```python
from build123d import *

# Parameters (mm, degrees)
F0_W         = 100
F0_H         = 100
F1_DEPTH     = 20
F2_T         = -1.6
F3_R         = 5
F4_T1_DEPTH  = 13.4
F4_S5_W      = 5
F4_S5_H      = 5
F4_T6_DEPTH  = 5
F4_S11_W     = 5
F4_S11_H     = 5
F4_T12_DEPTH = 5
F4_S17_W     = 5
F4_S17_H     = 5
F4_T18_DEPTH = 5
F4_S23_W     = 5
F4_S23_H     = 5
F4_T24_DEPTH = 5
F5_R         = 5
F6_R         = 5


# Not quite as in the source:
# - a fillet or chamfer that OpenCascade refuses, or shapes differently, is made with other operations: its cross-section is extruded or revolved along the edge and cut away or added


with BuildPart() as f1:
    # F0 (on Top) → F1 (new body)
    with BuildSketch(Plane.XY):
        Rectangle(F0_W, F0_H)
    extrude(amount=F1_DEPTH)

    # F2
    f2_openings = [f1.faces().sort_by_distance(p)[0] for p in [
        (0, 0, 20),
    ]]
    offset(amount=F2_T, openings=f2_openings)

    # F3
    f3_edges = [f1.edges().sort_by_distance(p)[0] for p in [
        (-48.4, 0, 1.6),
        (0, 48.4, 1.6),
        (48.4, 0, 1.6),
        (0, -48.4, 1.6),
    ]]
    fillet(f3_edges, radius=F3_R)

    # F4: fillet of radius 5 on 8 edges, made by hand

    # F4_s2 → F4_t1 (join)
    with BuildSketch(Plane.XY.offset(6.6)):
        with BuildLine():
            ThreePointArc((43.4, 48.4), (46.9355339059, 46.9355339059), (48.4, 43.4))
            Line((48.4, 43.4), (48.4, 48.4))
            Line((48.4, 48.4), (43.4, 48.4))
        make_face()
        with BuildLine():
            ThreePointArc((48.4, -43.4), (46.9355339059, -46.9355339059), (43.4, -48.4))
            Line((43.4, -48.4), (48.4, -48.4))
            Line((48.4, -48.4), (48.4, -43.4))
        make_face()
        with BuildLine():
            ThreePointArc((-48.4, -43.4), (-46.9355339059, -46.9355339059), (-43.4, -48.4))
            Line((-43.4, -48.4), (-48.4, -48.4))
            Line((-48.4, -48.4), (-48.4, -43.4))
        make_face()
        with BuildLine():
            ThreePointArc((-43.4, 48.4), (-46.9355339059, 46.9355339059), (-48.4, 43.4))
            Line((-48.4, 43.4), (-48.4, 48.4))
            Line((-48.4, 48.4), (-43.4, 48.4))
        make_face()
    extrude(amount=F4_T1_DEPTH)


with BuildPart() as f4_tool4:
    # F4_s5 → F4_t6 (new body)
    with BuildSketch(Plane.XZ.offset(-43.4)):
        with Locations((45.9, 4.1)):
            Rectangle(F4_S5_W, F4_S5_H)
    extrude(amount=-F4_T6_DEPTH)

    # F4_s7 → F4_t8 (revolve, cut)
    with BuildSketch(Plane(origin=(43.4, 43.4, 6.6), x_dir=(-0.7071067812, 0, 0.7071067812), z_dir=(-0.7071067812, 0, -0.7071067812))):
        with BuildLine():
            ThreePointArc((0, -5), (5, 0), (0, 5))
            Line((0, 5), (0, -5))
        make_face()
    revolve(axis=Axis((43.4, 43.4, 6.6), (0, 1, 0)), mode=Mode.SUBTRACT)


with BuildPart() as f1_1:
    add(f1.part)

    # F4_t3: union F4_tool4
    add(f4_tool4.part)


with BuildPart() as f4_tool10:
    # F4_s11 → F4_t12 (new body)
    with BuildSketch(Plane.YZ.offset(43.4)):
        with Locations((-45.9, 4.1)):
            Rectangle(F4_S11_W, F4_S11_H)
    extrude(amount=F4_T12_DEPTH)

    # F4_s13 → F4_t14 (revolve, cut)
    with BuildSketch(Plane(origin=(43.4, -43.4, 6.6), x_dir=(0, 0.7071067812, 0.7071067812), z_dir=(0, 0.7071067812, -0.7071067812))):
        with BuildLine():
            ThreePointArc((0, -5), (5, 0), (0, 5))
            Line((0, 5), (0, -5))
        make_face()
    revolve(axis=Axis((43.4, -43.4, 6.6), (1, 0, 0)), mode=Mode.SUBTRACT)


with BuildPart() as f1_2:
    add(f1_1.part)

    # F4_t9: union F4_tool10
    add(f4_tool10.part)


with BuildPart() as f4_tool16:
    # F4_s17 → F4_t18 (new body)
    with BuildSketch(Plane.YZ.offset(-43.4)):
        with Locations((-45.9, 4.1)):
            Rectangle(F4_S17_W, F4_S17_H)
    extrude(amount=-F4_T18_DEPTH)

    # F4_s19 → F4_t20 (revolve, cut)
    with BuildSketch(Plane(origin=(-43.4, -43.4, 6.6), x_dir=(0, 0.7071067812, 0.7071067812), z_dir=(0, -0.7071067812, 0.7071067812))):
        with BuildLine():
            ThreePointArc((0, -5), (5, 0), (0, 5))
            Line((0, 5), (0, -5))
        make_face()
    revolve(axis=Axis((-43.4, -43.4, 6.6), (-1, 0, 0)), mode=Mode.SUBTRACT)


with BuildPart() as f1_3:
    add(f1_2.part)

    # F4_t15: union F4_tool16
    add(f4_tool16.part)


with BuildPart() as f4_tool22:
    # F4_s23 → F4_t24 (new body)
    with BuildSketch(Plane.XZ.offset(-43.4)):
        with Locations((-45.9, 4.1)):
            Rectangle(F4_S23_W, F4_S23_H)
    extrude(amount=-F4_T24_DEPTH)

    # F4_s25 → F4_t26 (revolve, cut)
    with BuildSketch(Plane(origin=(-43.4, 43.4, 6.6), x_dir=(0.7071067812, 0, 0.7071067812), z_dir=(-0.7071067812, 0, 0.7071067812))):
        with BuildLine():
            ThreePointArc((0, -5), (5, 0), (0, 5))
            Line((0, 5), (0, -5))
        make_face()
    revolve(axis=Axis((-43.4, 43.4, 6.6), (0, 1, 0)), mode=Mode.SUBTRACT)


with BuildPart() as f1_4:
    add(f1_3.part)

    # F4_t21: union F4_tool22
    add(f4_tool22.part)

    # F5
    f5_edges = [f1_4.edges().sort_by_distance(p)[0] for p in [
        (50, -50, 10),
        (-50, -50, 10),
        (-50, 50, 10),
        (50, 50, 10),
    ]]
    fillet(f5_edges, radius=F5_R)

    # F6
    f6_edges = [f1_4.edges().sort_by_distance(p)[0] for p in [
        (-50, 0, 0),
        (0, 50, 0),
        (-48.535534, 48.535534, 0),
        (48.535534, 48.535534, 0),
        (50, 0, 0),
        (48.535534, -48.535534, 0),
        (0, -50, 0),
        (-48.535534, -48.535534, 0),
    ]]
    fillet(f6_edges, radius=F6_R)


solid = f1_4.part
```
Build history of the part. All positions in model axes, mm. A direction names the side the tool comes from. Round coordinates to 2 decimals unless told otherwise and drop trailing zeros. Write each loop counter-clockwise with the first axis right and the second up, starting at its lowest first coordinate (ties: lowest second). Pieces come first, ordered by that corner, then holes. Notation, with made-up numbers: (12.5, 6.25) - (30.5, 6.25) arc R33 cw to (30.5, 38.25) - close; hole circle Ø10 at (-29.5, -14). An arc over 180 degrees is marked (long way). Write each question's results on one line, items separated by ' | '. Start each with the question number.
Item 1: Saw through at B-B (y = -41). Write the cut outline in (x, z), and give its area (3 significant figures).
Item 2: Wall check: L1, parallel to Y at x = -28.5, z = 18.25; L2, parallel to Z at x = -39, y = 3. Give the ranges that are in metal, low to high. Write a range as [from, to].
Item 3: Which spindle directions (+Z, -Z, +X, -X, +Y, -Y) get a long thin tool onto all of the face, cutting with end or side? Do faces 1 (the face through (-46.97, -46.9, 13.21)), 2 (the face through (-1, 50, 12)). Say none if no direction does.
Item 4: Mould opens along Y. For faces 3 (the face through (-1, 1, 0)), 4 (the face through (-1, -50, 12)), 5 (the face through (-46.97, 0.61, 3.1)), 6 (the face through (-48.4, -1, 13)) say: pulls with the +Y half, pulls with the -Y half, needs draft (parallel to the pull), parting line crosses it, or undercut.
Item 5: Saw through at A-A (z = 9.5). Write the cut outline in (x, y), and give its area (3 significant figures).
Item 6: Drop a flat-ended pin along its axis: P1, Ø1, axis at x = -7, z = 3.5, coming from the -Y side. Give the stop position or say it passes through.
Results are:
1) outline: (-50, 5) arc R5 ccw to (-45, 0) - (45, 0) arc R5 ccw to (50, 5) - (50, 20) - (48.4, 20) - (48.4, 6.6) arc R5 cw to (43.4, 1.6) - (-43.4, 1.6) arc R5 cw to (-48.4, 6.6) - (-48.4, 20) - (-50, 20) - close | area: 219 mm²
2) L1: y = [-50, -48.4], [48.4, 50] | L2: z = [0, 1.6]
3) face 1: +Z | face 2: +Z, -Z, +X, -X, +Y
4) face 3: needs draft | face 4: pulls with the -Y half | face 5: undercut | face 6: undercut
5) outline: (-50, -45) arc R5 ccw to (-45, -50) - (45, -50) arc R5 ccw to (50, -45) - (50, 45) arc R5 ccw to (45, 50) - (-45, 50) arc R5 ccw to (-50, 45) - close; hole (-48.4, -43.4) arc R5 ccw to (-43.4, -48.4) - (43.4, -48.4) arc R5 ccw to (48.4, -43.4) - (48.4, 43.4) arc R5 ccw to (43.4, 48.4) - (-43.4, 48.4) arc R5 ccw to (-48.4, 43.4) - close | area: 630 mm²
6) P1: stops at y = -49.9
